Geometry check sheet. Reference: drawing and pictorial views, mm from the part's lowest x, y, z. A direction names the side the tool comes from. Coordinates: 2 decimals unless noted, no trailing zeros. Loops run counter-clockwise (first coordinate to the right, second up) from the corner with the lowest first, then second, coordinate; pieces in that order, holes last. Notation, with made-up numbers: (-19.75, 8) -> (11.25, 8) arc R25 cw to (11.25, 47) -> close; hole circle Ø10 at (64.5, 32). An arc over 180 degrees is marked (long way). Use CSV: the item, a comma, the result in double quotes.
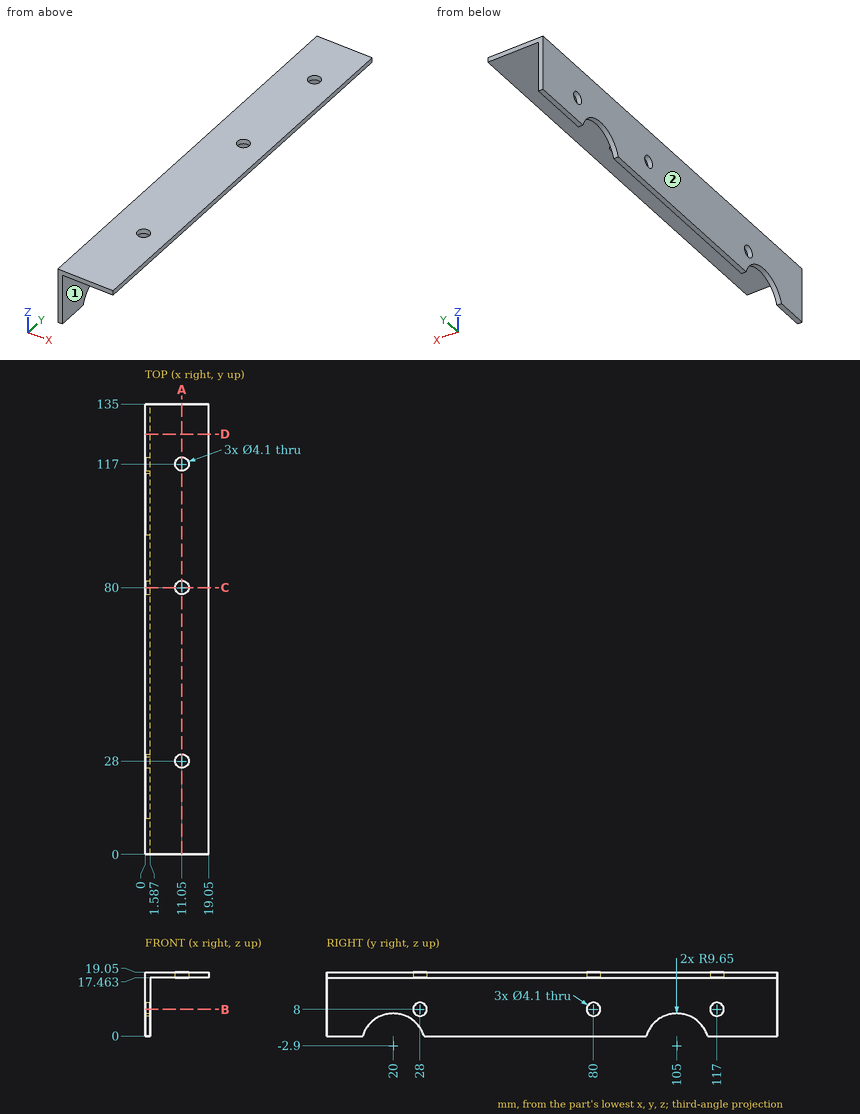
1) Go/stop test with flat-tipped pins: pin 1 Ø3.5 at (x, y) = (11.05, 28) entering from -Z; pin 2 Ø10 at (x, z) = (9, 16) entering from +Y; pin 3 Ø5 at (x, y) = (13.5, 73) entering from -Z; pin 4 Ø4 at (y, z) = (97, 8.5) entering from +X. Record where each tip stops, or that it passes through.
Answer below:
pin 1,"passes through"
pin 2,"stops at y = 135"
pin 3,"stops at z = 17.46"
pin 4,"stops at x = 1.59"
2) Cross-section at A-A on x = 11.05. Record the boundary of the cut face in (y, z), and give its area (3 significant figures).
Answer below:
outline,"(0, 17.46) -> (25.95, 17.46) -> (25.95, 19.05) -> (0, 19.05) -> close; (30.05, 17.46) -> (77.95, 17.46) -> (77.95, 19.05) -> (30.05, 19.05) -> close; (82.05, 17.46) -> (114.95, 17.46) -> (114.95, 19.05) -> (82.05, 19.05) -> close; (119.05, 17.46) -> (135, 17.46) -> (135, 19.05) -> (119.05, 19.05) -> close"
area,"195 mm²"
3) Access from +Z, -Z, +X, -X, +Y, -Y to the whole of each face (thin tool, end or side, straight path). Record for the marked faces 1 and 2.
Answer below:
face 1,"-Z, +X, +Y, -Y"
face 2,"+Z, -Z, -X, +Y, -Y"
4) Cross-section at D-D on y = 126. Record the boundary of the cut face in (x, z).
Answer below:
outline,"(0, 0) -> (1.59, 0) -> (1.59, 17.46) -> (19.05, 17.46) -> (19.05, 19.05) -> (0, 19.05) -> close"
5) Cross-section at C-C on y = 80. Record the boundary of the cut face in (x, z).
Answer below:
outline,"(0, 0) -> (1.59, 0) -> (1.59, 5.95) -> (0, 5.95) -> close; (0, 10.05) -> (1.59, 10.05) -> (1.59, 17.46) -> (9, 17.46) -> (9, 19.05) -> (0, 19.05) -> close; (13.1, 17.46) -> (19.05, 17.46) -> (19.05, 19.05) -> (13.1, 19.05) -> close"
6) Cross-section at B-B on z = 8. Record the boundary of the cut face in (x, y), and give its area (3 significant figures).
Answer below:
outline,"(0, 0) -> (1.59, 0) -> (1.59, 25.95) -> (0, 25.95) -> close; (0, 30.05) -> (1.59, 30.05) -> (1.59, 77.95) -> (0, 77.95) -> close; (0, 82.05) -> (1.59, 82.05) -> (1.59, 114.95) -> (0, 114.95) -> close; (0, 119.05) -> (1.59, 119.05) -> (1.59, 135) -> (0, 135) -> close"
area,"195 mm²"
7) Thickness scan on line 1 along Y through (x, z) = (11.05, 17.95); line 2 along X through (y, z) = (69, 16.5); line 3 along Z through (x, y) = (5, 44). Record the ranges inside material, lowest first. Write a range as from..to.
Answer below:
line 1,"y = 0..25.95, 30.05..77.95, 82.05..114.95, 119.05..135"
line 2,"x = 0..1.59"
line 3,"z = 17.46..19.05"
